CAD build for the part. Positions are in the model's coordinates, mm. Face numbers are marked on the shaded views. Round coordinates to 2 decimals unless told otherwise and drop trailing zeros. Loops run counter-clockwise (first coordinate to the right, second up) from the corner with the lowest first, then second, coordinate; pieces in that order, holes last.
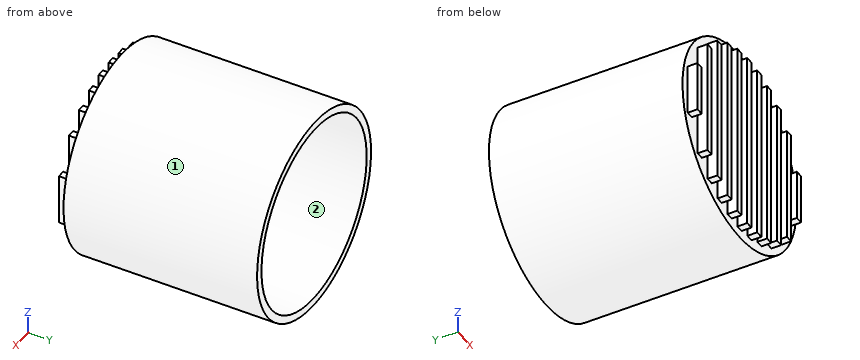
```python
from build123d import *

# Parameters (mm, degrees)
SKETCH1_R           = 38.1
BOSS_EXTRUDE1_DEPTH = 76.2
SHELL2_T            = 3.175
SKETCH2_W           = 3
SKETCH2_H           = 75
SKETCH2_H_2         = 48.033738144
SKETCH2_H_3         = 61.308726948
SKETCH2_H_4         = 69.24998195
SKETCH2_H_5         = 73.60461942
BOSS_EXTRUDE2_DEPTH = 4


with BuildPart() as part:
    # Sketch1 → Boss-Extrude1 (new body)
    with BuildSketch(Plane(origin=(0, 0, 0), x_dir=(1, 0, 0), z_dir=(0, 1, 0))):
        with Locations(Location((0, 0, 0), (0, 0, 90))):
            Circle(SKETCH1_R)
    extrude(amount=BOSS_EXTRUDE1_DEPTH)

    # Shell2
    shell2_openings = [part.faces().sort_by_distance(p)[0] for p in [
        (0, 76.2, 0),
    ]]
    offset(amount=SHELL2_T, openings=shell2_openings, kind=Kind.INTERSECTION)

    # Sketch2 → Boss-Extrude2 (add)
    with BuildSketch(Plane.XZ.offset(3.175)):
        Rectangle(SKETCH2_W, SKETCH2_H)
        Polygon((-34.5, -10.5), (-34.5, 0), (-34.5, 10.5), (-37.5, 10.5), (-37.5, -10.5), align=None)
        with Locations((-28.8, 0)):
            Rectangle(SKETCH2_W, SKETCH2_H_2)
        with Locations((-21.6, 0)):
            Rectangle(SKETCH2_W, SKETCH2_H_3)
        with Locations((-14.4, 0)):
            Rectangle(SKETCH2_W, SKETCH2_H_4)
        with Locations((-7.2, 0)):
            Rectangle(SKETCH2_W, SKETCH2_H_5)
        Polygon((8.7, -36.80230971), (8.7, 0), (8.7, 36.80230971), (5.7, 36.80230971), (5.7, -36.80230971), align=None)
        with Locations((14.4, 0)):
            Rectangle(SKETCH2_W, SKETCH2_H_4)
        with Locations((21.6, 0)):
            Rectangle(SKETCH2_W, SKETCH2_H_3)
        with Locations((28.8, 0)):
            Rectangle(SKETCH2_W, SKETCH2_H_2)
        Polygon((37.5, -10.5), (37.5, 10.5), (34.5, 10.5), (34.5, 0), (34.5, -10.5), align=None)
    extrude(amount=BOSS_EXTRUDE2_DEPTH)


solid = part.part
```
Item 1: Cut at C-C, the plane z = 32. Give the cut face in (x, y) (3 decimals), plus the area to 3 significant figures.
Answers follow:
outline: (-26.07, -3.175) - (-15.9, -3.175) - (-15.9, -7.175) - (-12.9, -7.175) - (-12.9, -3.175) - (-8.7, -3.175) - (-8.7, -7.175) - (-5.7, -7.175) - (-5.7, -3.175) - (-1.5, -3.175) - (-1.5, -7.175) - (1.5, -7.175) - (1.5, -3.175) - (5.7, -3.175) - (5.7, -7.175) - (8.7, -7.175) - (8.7, -3.175) - (12.9, -3.175) - (12.9, -7.175) - (15.9, -7.175) - (15.9, -3.175) - (26.07, -3.175) - (26.07, 76.2) - (20.679, 76.2) - (20.679, 0) - (-20.679, 0) - (-20.679, 76.2) - (-26.07, 76.2) - close
area: 1,050 mm2
Item 2: Probe line 1 (X direction, y = 44, z = 0) (3 decimals); line 2 (Y direction, x = 3.5, z = -14) (3 decimals); line 3 (Z direction, x = -12.5, y = 29.5). List the from-to ranges inside material, lowest first.
Answers follow:
line 1: x = -41.275 to -38.1, 38.1 to 41.275
line 2: y = -3.175 to 0
line 3: z = -39.34 to -35.99, 35.99 to 39.34
Item 3: Cut at A-A, the plane x = 0. Give the cut face in (y, z) (3 decimals).
Answers follow:
outline: (-7.175, -37.5) - (-3.175, -37.5) - (-3.175, -41.275) - (76.2, -41.275) - (76.2, -38.1) - (0, -38.1) - (0, 38.1) - (76.2, 38.1) - (76.2, 41.275) - (-3.175, 41.275) - (-3.175, 37.5) - (-7.175, 37.5) - close
Item 4: Flat gauge pins, fed straight in: P1, Ø4, axis at y = 66.5, z = 17, coming from the +X side; P2, Ø1.2, axis at y = -6, z = 15, coming from the +X side; P3, Ø6, axis at y = 50.5, z = -18, coming from the -X side. Where does each tip first touch, or does it go through?
Answers follow:
P1: stops at x = 38.45
P2: stops at x = 30.3
P3: stops at x = -38.45
Item 5: Two-plate mould, pull along Z, no slides. Class the marked faces 1 and 2: released by +Z, released by -Z, zero draft, split by the parting line, or undercut.
Answers follow:
face 1: split by the parting line
face 2: undercut
Item 6: Cut at B-B, the plane y = 16. Give the cut face in (x, z) (3 decimals).
Answers follow:
outline: circle Ø82.55 at (0, 0); hole circle Ø76.2 at (0, 0)
Item 7: Cut at D-D, the plane x = -11.5. Give the cut face in (y, z) (3 decimals).
Answers follow:
outline: (-3.175, -39.641) - (76.2, -39.641) - (76.2, -36.323) - (0, -36.323) - (0, 36.323) - (76.2, 36.323) - (76.2, 39.641) - (-3.175, 39.641) - close
